Model file for the job. Use its own axes, mm. Face numbers are marked on the shaded views. A direction names the side the tool comes from. Coordinates: 2 decimals unless noted, no trailing zeros. Write item = value, one per line. Start each with the question number.
Q1. 3-axis set-ups, long thin cutter, end or side, ignore diameter. For the marked faces 4, 5, 6 and 7: which of +Z, -Z, +X, -X, +Y, -Y reach the whole face in a straight line?
Q2. Flat gauge pins, fed straight in: pin 1 (1.5 mm diameter, centred on y = -6, z = -17.5, fed in from -X); pin 2 (2.5 mm diameter, centred on x = 0, y = 20.64, fed in from -Z) (3 decimals); pin 3 (12 mm diameter, centred on x = -5, z = -12.5, fed in from +Y); pin 4 (3 mm diameter, centred on y = 6, z = -14, fed in from -X). Where does each tip first touch, or does it go through?
Q3. Wall check: line 1 (Y direction, x = -0.5, z = -4.75) (3 decimals); line 2 (Y direction, x = 0, z = -1.1) (1 decimal); line 3 (Z direction, x = 4.75, y = -6) (3 decimals). Give the ranges that are in metal, low to high. Write a range as from..to.
Q4. Cut at A-A, the plane x = 0. Give the number of separate pieces and of enclosed holes in the cut face, plus the area to 4 significant figures.
Q5. Mould opens along Y. For the marked faces 1, 2 and 3 say: +Y half, -Y half, draft (parallel to the pull), parting line (faces both ways), or undercut.
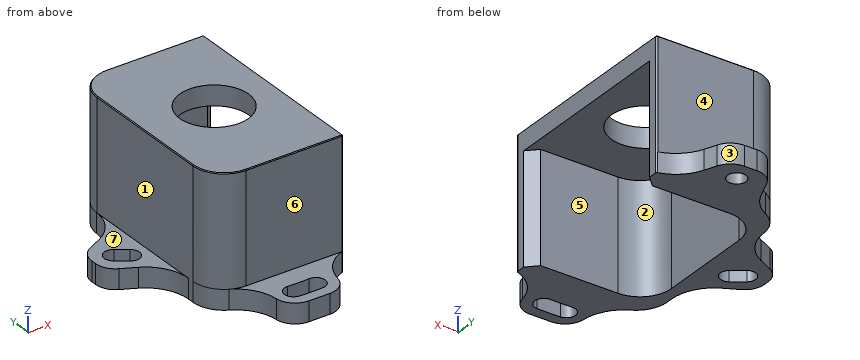
from build123d import *

# Parameters (mm, degrees)
BOSS_EXTRUDE1_DEPTH   = 9.525
SKETCH2_R             = 5.5245
CUT_EXTRUDE1_DEPTH    = 35.200748661
SKETCH11_W            = 17.653
SKETCH11_H            = 9.525
CUT_EXTRUDE4_DEPTH    = 38.971938112
F_4_CLEARANCE_HOLE1_D = 2.9464
CUT_EXTRUDE5_DEPTH    = 33.365321472
BOSS_EXTRUDE2_DEPTH   = 1.5875
SKETCH16_W            = 9.525
SKETCH16_H            = 50.8
BOSS_EXTRUDE3_DEPTH   = 3.175
FILLET1_R             = 5.0165
CUT_EXTRUDE6_DEPTH    = 38.184604546
FILLET3_R             = 0.254
CHAMFER1_SIZE         = 0.127
CHAMFER2_SIZE         = 1.5875
SKETCH18_OUTSIDE_W    = 44.691
SKETCH18_OUTSIDE_H    = 65.328
CUT_EXTRUDE7_DEPTH    = 38.184604546
FILLET5_START         = -20.828
FILLET5_DEPTH         = 3.175
FILLET6_R             = 3.175


with BuildPart() as part:
    # Sketch1 → Boss-Extrude1 (new, symmetric)
    with BuildSketch(Plane(origin=(0, 0, 0), x_dir=(0, 0, -1), z_dir=(1, 0, 0))):
        Polygon((0, 25.4), (0, -25.4), (20.828, -25.4), (20.828, -12.7), (3.175, -12.7), (3.175, 12.7), (20.828, 12.7), (20.828, 25.4), align=None)
    extrude(amount=BOSS_EXTRUDE1_DEPTH, both=True)

    # Sketch2 → Cut-Extrude1 (cut, through all)
    with BuildSketch(Plane.XY):
        Circle(SKETCH2_R)
    extrude(amount=-CUT_EXTRUDE1_DEPTH, mode=Mode.SUBTRACT)

    # Sketch11 → Cut-Extrude4 (cut, through all)
    with BuildSketch(Plane(origin=(9.525, 0, 0), x_dir=(0, 0, -1), z_dir=(1, 0, 0))):
        with Locations((8.8265, 20.6375)):
            Rectangle(SKETCH11_W, SKETCH11_H)
    cut_extrude4 = extrude(amount=-CUT_EXTRUDE4_DEPTH, mode=Mode.SUBTRACT)

    # #4 Clearance Hole1 (through all)
    with Locations(Plane.XY.offset(-17.653)):
        with Locations((0, 20.6375)):
            Hole(F_4_CLEARANCE_HOLE1_D / 2)

    # Mirror1: Cut-Extrude4 across plane
    add(cut_extrude4.mirror(Plane.ZX), mode=Mode.SUBTRACT)

    # Sketch14 → Cut-Extrude5 (cut, through all)
    with BuildSketch(Plane.XY.offset(-17.653)):
        with BuildLine():
            ThreePointArc((-1.864650295, -22.070013186), (0, -22.1107), (1.864650295, -22.070013186))
            ThreePointArc((1.864650295, -22.070013186), (3.272188054, -20.533955264), (1.736130132, -19.126417506))
            ThreePointArc((1.736130132, -19.126417506), (0, -19.1643), (-1.736130132, -19.126417506))
            ThreePointArc((-1.736130132, -19.126417506), (-3.272188054, -20.533955264), (-1.864650295, -22.070013186))
        make_face()
    extrude(amount=-CUT_EXTRUDE5_DEPTH, mode=Mode.SUBTRACT)

    # Sketch15 → Boss-Extrude2 (add)
    with BuildSketch(Plane.ZY.offset(9.525)):
        Polygon((-20.828, 12.7), (-20.828, 25.4), (-17.653, 25.4), (-17.653, 15.875), (0, 15.875), (0, -15.875), (-17.653, -15.875), (-17.653, -25.4), (-20.828, -25.4), (-20.828, -12.7), align=None)
    extrude(amount=BOSS_EXTRUDE2_DEPTH)

    # Sketch16 → Boss-Extrude3 (add)
    with BuildSketch(Plane.XY.offset(-17.653)):
        with Locations((-15.875, 0)):
            Rectangle(SKETCH16_W, SKETCH16_H)
    extrude(amount=-BOSS_EXTRUDE3_DEPTH)

    # Fillet1
    fillet1_edges = [part.edges().sort_by_distance(p)[0] for p in [
        (-9.525, 12.7, -12.0015),
        (-11.1125, -15.875, -8.8265),
        (-11.1125, 15.875, -8.8265),
        (-9.525, -12.7, -12.0015),
    ]]
    fillet(fillet1_edges, radius=FILLET1_R)

    # Sketch17 → Cut-Extrude6 (cut, through all)
    with BuildSketch(Plane.XY.offset(-17.653)):
        with BuildLine():
            ThreePointArc((-16.603528504, -0.49285067), (-15.666032673, -1.196975), (-14.698715658, -1.859536166))
            ThreePointArc((-14.698715658, -1.859536166), (-12.659629074, -1.432028992), (-13.087136248, 0.607057592))
            ThreePointArc((-13.087136248, 0.607057592), (-13.94839582, 1.196975), (-14.783103829, 1.823898553))
            ThreePointArc((-14.783103829, 1.823898553), (-16.851690778, 1.575736279), (-16.603528504, -0.49285067))
        make_face()
    extrude(amount=-CUT_EXTRUDE6_DEPTH, mode=Mode.SUBTRACT)

    # Fillet3
    fillet3_edges = [part.edges().sort_by_distance(p)[0] for p in [
        (9.525, 15.875, -8.8265),
        (9.525, -15.875, -8.8265),
    ]]
    fillet(fillet3_edges, radius=FILLET3_R)

    # Chamfer1
    chamfer1_edges = [part.edges().sort_by_distance(p)[0] for p in [
        (-11.1125, 0, 0),
        (1.5875, 15.875, 0),
        (1.5875, -15.875, 0),
        (-9.643201168, -14.405701168, 0),
        (-9.643201168, 14.405701168, 0),
        (9.525, 0, 0),
        (9.450605122, -15.800605122, 0),
        (9.450605122, 15.800605122, 0),
    ]]
    chamfer(chamfer1_edges, length=CHAMFER1_SIZE)

    # Chamfer2
    chamfer2_edges = [part.edges().sort_by_distance(p)[0] for p in [
        (9.525, -12.7, -12.0015),
        (9.525, 12.7, -12.0015),
    ]]
    chamfer(chamfer2_edges, length=CHAMFER2_SIZE)

    # Sketch18 outside → Cut-Extrude7 (cut, through all)
    with BuildSketch(Plane.XY.offset(-17.653)):
        with Locations((-5.5565, 0)):
            Rectangle(SKETCH18_OUTSIDE_W, SKETCH18_OUTSIDE_H)
        with BuildLine():
            Line((9.525, 15.621), (9.525, -15.621))
            ThreePointArc((9.525, -15.621), (9.450605122, -15.800605122), (9.271, -15.875))
            Line((9.271, -15.875), (4.7625, -15.875))
            Line((4.7625, -15.875), (4.7625, -23.8125))
            Line((4.7625, -23.8125), (-4.7625, -23.8125))
            Line((-4.7625, -23.8125), (-4.7625, -15.875))
            Line((-4.7625, -15.875), (-6.096, -15.875))
            ThreePointArc((-6.096, -15.875), (-9.643201168, -14.405701168), (-11.1125, -10.8585))
            Line((-11.1125, -10.8585), (-11.1125, -5.684476059))
            Line((-11.1125, -5.684476059), (-18.868316167, -1.715726059))
            Line((-18.868316167, -1.715726059), (-18.868316167, 3.046773941))
            Line((-18.868316167, 3.046773941), (-11.1125, 7.015523941))
            Line((-11.1125, 7.015523941), (-11.1125, 10.8585))
            ThreePointArc((-11.1125, 10.8585), (-9.730137534, 14.316579906), (-6.344906405, 15.868821133))
            Line((-6.344906405, 15.868821133), (-3.175, 23.8125))
            Line((-3.175, 23.8125), (3.175, 23.8125))
            Line((3.175, 23.8125), (6.360346812, 15.875))
            Line((6.360346812, 15.875), (9.271, 15.875))
            ThreePointArc((9.271, 15.875), (9.450605122, 15.800605122), (9.525, 15.621))
        make_face(mode=Mode.SUBTRACT)
    extrude(amount=-CUT_EXTRUDE7_DEPTH, mode=Mode.SUBTRACT)

    # Fillet5: read off the stored shape, not the designer's step
    # Fillet5 outline → Fillet5 (add)
    with BuildSketch(Plane.XY.offset(FILLET5_START)):
        with BuildLine():
            Line((-6.344906405, 15.868821133), (-5.141439076, 18.884669795))
            ThreePointArc((-5.141439076, 18.884669795), (-6.439586705, 16.809867774), (-8.383629538, 15.323029465))
            ThreePointArc((-8.383629538, 15.323029465), (-7.393295565, 15.704353533), (-6.344906405, 15.868821133))
        make_face()
        with BuildLine():
            Line((4.728452297, 19.941484272), (6.360346812, 15.875))
            Line((6.360346812, 15.875), (9.271, 15.875))
            ThreePointArc((9.271, 15.875), (9.303812086, 15.872871727), (9.336074306, 15.866522574))
            ThreePointArc((9.336074306, 15.866522574), (6.549781647, 17.358453978), (4.728452297, 19.941484272))
        make_face()
        with BuildLine():
            Line((9.271, -15.875), (4.7625, -15.875))
            Line((4.7625, -15.875), (4.7625, -22.333703908))
            ThreePointArc((4.7625, -22.333703908), (6.027219419, -18.365407505), (9.354910714, -15.860739425))
            ThreePointArc((9.354910714, -15.860739425), (9.313556938, -15.871409478), (9.271, -15.875))
        make_face()
        with BuildLine():
            ThreePointArc((-6.096, -15.875), (-7.297950449, -15.728878565), (-8.429879679, -15.299026759))
            ThreePointArc((-8.429879679, -15.299026759), (-5.750515411, -17.823432924), (-4.7625, -21.369620302))
            Line((-4.7625, -21.369620302), (-4.7625, -15.875))
            Line((-4.7625, -15.875), (-6.096, -15.875))
        make_face()
        with BuildLine():
            Line((-11.1125, -9.878885048), (-11.1125, -5.684476059))
            Line((-11.1125, -5.684476059), (-14.846436435, -3.773773186))
            ThreePointArc((-14.846436435, -3.773773186), (-12.119987547, -6.300663697), (-11.1125, -9.878885048))
        make_face()
        with BuildLine():
            ThreePointArc((-11.1125, 10.8585), (-11.11194212, 10.933312395), (-11.110268606, 11.008108151))
            ThreePointArc((-11.110268606, 11.008108151), (-12.168719233, 7.547562085), (-14.841154527, 5.107523888))
            Line((-14.841154527, 5.107523888), (-11.1125, 7.015523941))
            Line((-11.1125, 7.015523941), (-11.1125, 10.8585))
        make_face()
    extrude(amount=FILLET5_DEPTH)

    # Fillet6
    fillet6_edges = [part.edges().sort_by_distance(p)[0] for p in [
        (-3.175, 23.8125, -19.2405),
        (3.175, 23.8125, -19.2405),
        (4.7625, -23.8125, -19.2405),
        (-4.7625, -23.8125, -19.2405),
        (-18.868316167, 3.046773941, -19.2405),
        (-18.868316167, -1.715726059, -19.2405),
    ]]
    fillet(fillet6_edges, radius=FILLET6_R)


solid = part.part
Here are the results:
q1.face_4 = +Z, +X, -X, +Y
q1.face_5 = -Z, +X
q1.face_6 = +Z, +X, -X, -Y
q1.face_7 = +Z, -X, +Y, -Y
q2.pin_1 = -12.9
q2.pin_2 = through
q2.pin_3 = 23.68
q2.pin_4 = -11.11
q3.line_1 = -15.875..-12.7, 12.7..15.875
q3.line_2 = -15.9..-5.5, 5.5..15.9
q3.line_3 = -3.175..0
q4.separate_pieces = 4
q4.enclosed_holes = 0
q4.area = 209.5 mm²
q5.face_1 = draft
q5.face_2 = undercut
q5.face_3 = +Y half
